Build history of the part. All positions in model axes, mm. Face numbers are marked on the shaded views. A direction names the side the tool comes from. Give positions to 0.01 mm unless a question says otherwise; leave off trailing zeros. Write each loop counter-clockwise with the first axis right and the second up, starting at its lowest first coordinate (ties: lowest second). Pieces come first, ordered by that corner, then holes. Notation, with made-up numbers: (-31.5, 9.25) -> (-26.5, 9.25) arc R22 ccw to (-26.5, 37.25) -> close; hole circle Ø3 at (73, 57). An arc over 180 degrees is marked (long way). Put each result on its own line as item: value.
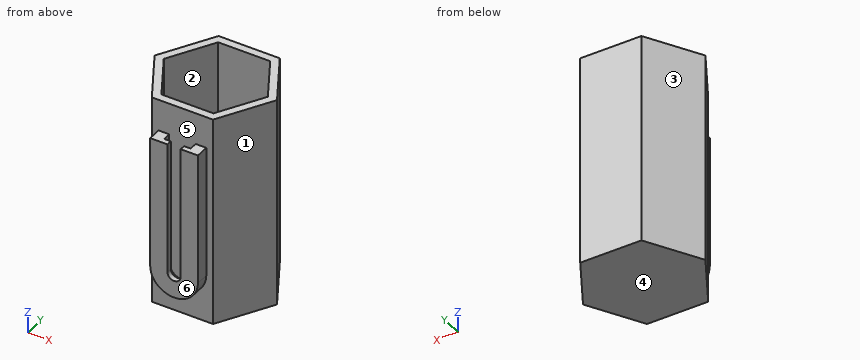
from build123d import *

# Parameters (mm, degrees)
F1_DEPTH = 80
F3_DEPTH = 5
F5_DEPTH = 3
F7_DEPTH = 2


with BuildPart() as f1:
    # F0 (on Top) → F1 (new body)
    with BuildSketch(Plane.XY):
        Polygon((11.547005, 20), (-11.547005, 20), (-23.094011, 0), (-11.547005, -20), (11.547005, -20), (23.094011, 0), align=None)
        Polygon((-9.814955, -17), (-19.629909, 0), (-9.814955, 17), (9.814955, 17), (19.629909, 0), (9.814955, -17), align=None, mode=Mode.SUBTRACT)
    extrude(amount=F1_DEPTH)

    # F2 (on Top) → F3 (join)
    with BuildSketch(Plane.XY):
        Polygon((11.547005, 20), (-11.547005, 20), (-23.094011, 0), (-11.547005, -20), (11.547005, -20), (23.094011, 0), align=None)
    extrude(amount=F3_DEPTH)

    # F4 (on face) → F5 (join)
    with BuildSketch(Plane.XZ.offset(20)):
        with BuildLine():
            Line((-5, 18), (-5, 68))
            Line((-5, 68), (-9, 68))
            Line((-9, 68), (-9, 18))
            ThreePointArc((-9, 18), (0, 9), (9, 18))
            Line((9, 18), (9, 68))
            Line((9, 68), (5, 68))
            Line((5, 68), (5, 18))
            ThreePointArc((5, 18), (0, 13), (-5, 18))
        make_face()
    extrude(amount=F5_DEPTH)

    # F6 (on face) → F7 (join)
    with BuildSketch(Plane.XZ.offset(23)):
        with BuildLine():
            Line((-2.5, 68), (-9, 68))
            Line((-9, 68), (-9, 18))
            ThreePointArc((-9, 18), (0, 9), (9, 18))
            Line((9, 18), (9, 68))
            Line((9, 68), (2.5, 68))
            Line((2.5, 68), (2.5, 18))
            ThreePointArc((2.5, 18), (0, 15.5), (-2.5, 18))
            Line((-2.5, 18), (-2.5, 68))
        make_face()
    extrude(amount=F7_DEPTH)


solid = f1.part
1) Slice it at B-B (x = 0). Write the cut outline in (y, z), plus the area to 3 significant figures.
Filled sheet:
outline: (-25, 9) -> (-20, 9) -> (-20, 0) -> (20, 0) -> (20, 80) -> (17, 80) -> (17, 5) -> (-17, 5) -> (-17, 80) -> (-20, 80) -> (-20, 13) -> (-23, 13) -> (-23, 15.5) -> (-25, 15.5) -> close
area: 675 mm2
2) Tool access for the marked faces 1 and 2: list every direction of +Z, -Z, +X, -X, +Y, -Y with a clear straight run to the whole face (end or side of a thin tool).
Filled sheet:
face 1: +Z, -Z, +X, -Y
face 2: +Z
3) Pin check, flat tips, straight feed: pin 1 (5.5 mm diameter, centred on y = -23.5, z = 52.5, fed in from -X); pin 2 (1 mm diameter, centred on y = -23.5, z = 49.5, fed in from +X); pin 3 (5 mm diameter, centred on x = 14, z = 28, fed in from -Y). Stop position of each tip, or through.
Filled sheet:
pin 1: x = -9
pin 2: x = 9
pin 3: y = -20
4) Slice it at D-D (z = 71). Write the cut outline in (x, y).
Filled sheet:
outline: (-23.09, 0) -> (-11.55, -20) -> (11.55, -20) -> (23.09, 0) -> (11.55, 20) -> (-11.55, 20) -> close; hole (-19.63, 0) -> (-9.81, -17) -> (9.81, -17) -> (19.63, 0) -> (9.81, 17) -> (-9.81, 17) -> close
5) Slice it at A-A (z = 21). Write the cut outline in (x, y), plus the area to 3 significant figures.
Filled sheet:
outline: (-23.09, 0) -> (-11.55, -20) -> (-9, -20) -> (-9, -25) -> (-2.5, -25) -> (-2.5, -23) -> (-5, -23) -> (-5, -20) -> (5, -20) -> (5, -23) -> (2.5, -23) -> (2.5, -25) -> (9, -25) -> (9, -20) -> (11.55, -20) -> (23.09, 0) -> (11.55, 20) -> (-11.55, 20) -> close; hole (-19.63, 0) -> (-9.81, -17) -> (9.81, -17) -> (19.63, 0) -> (9.81, 17) -> (-9.81, 17) -> close
area: 435 mm2
6) Slice it at C-C (y = 3.5). Write the cut outline in (x, z).
Filled sheet:
outline: (-21.07, 0) -> (21.07, 0) -> (21.07, 80) -> (17.61, 80) -> (17.61, 5) -> (-17.61, 5) -> (-17.61, 80) -> (-21.07, 80) -> close
7) Wall check: L1, parallel to Y at x = 4, z = 61; L2, parallel to Z at x = 6, y = -6; L3, parallel to X at y = 15, z = 38.5. Give the ranges that are in metal, low to high.
Filled sheet:
L1: -25 to -23, -20 to -17, 17 to 20
L2: 0 to 5
L3: -14.43 to -10.97, 10.97 to 14.43
8) Pull direction Y, two halves, no side cores. Call the marked faces 3, 4, 5 and 6: released by +Y, released by -Y, zero draft, split by the parting line, or undercut.
Filled sheet:
face 3: released by +Y
face 4: zero draft
face 5: undercut
face 6: released by -Y
